Work out the finished part from the listing and answer in its coordinate system (mm). Round coordinates to 2 decimals unless told otherwise and drop trailing zeros. Order: outer loops, then holes, each group sorted by start corner. A loop starts at its lowest first (then second) coordinate and runs counter-clockwise, first axis right, second up. Notation, with made-up numbers: (60.25, -6.75) - (83.25, -6.75) arc R5 cw to (83.25, 1.25) - close; hole circle Ø11 at (11.5, 71.25). An arc over 180 degrees is marked (long way). Use CSV: the item, a comma, the result in double quotes.
from build123d import *

# Parameters (mm, degrees)
F0_W     = 78.734032
F0_H     = 94.131536
F1_DEPTH = 85.5


with BuildPart() as f1:
    # F0 (on Front) → F1 (new body)
    with BuildSketch(Plane.XZ):
        Rectangle(F0_W, F0_H)
    extrude(amount=F1_DEPTH)


with BuildPart() as f3:
    # F2 (on Front) → F3 (revolve)
    with BuildSketch(Plane.XZ):
        with BuildLine():
            Line((0, 0), (0, 49.300977))
            ThreePointArc((0, 49.300977), (-49.300977, 0), (0, -49.300977))
            Line((0, -49.300977), (0, 0))
        make_face()
    revolve(axis=Axis((0, 0, 0), (0, 0, -1)))


with BuildPart() as f1_1:
    add(f1.part)

    # F4: intersect F3
    add(f3.part, mode=Mode.INTERSECT)


solid = f1_1.part
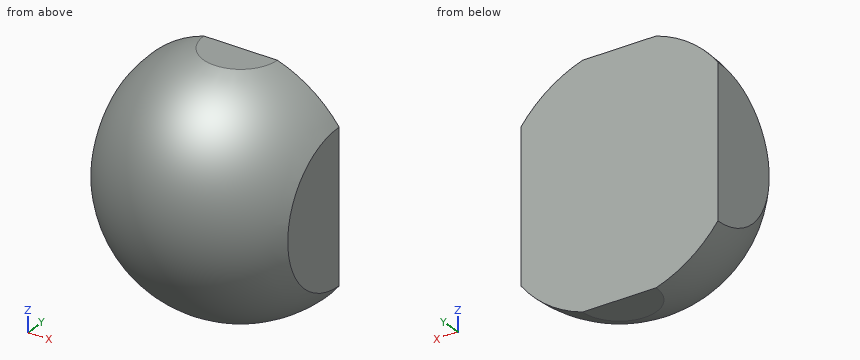
(1) Find section B-B (z = -15). Determine the outline of the cut face in (x, y), and give its area (3 significant figures).
Findings below:
outline,"(-39.37, -25.61) arc R46.96 ccw to (39.37, -25.61) - (39.37, 0) - (-39.37, 0) - close"
area,"3,200 mm²"
(2) Each of these flat-tipped pins is pushed along its axis until it touches: pin 1 (2 mm diameter, centred on y = -42, z = -0.5, fed in from +X); pin 2 (5 mm diameter, centred on x = 25.5, y = -29, fed in from -Z); pin 3 (2 mm diameter, centred on y = -35.5, z = 20.5, fed in from +X). Where does it stop, or does it pass through?
Findings below:
pin 1,"stops at x = 27.37"
pin 2,"stops at z = -33.56"
pin 3,"stops at x = 28.83"
(3) Find the intervals of material crossed by L1, parallel to Z at x = -20, y = -8; L2, parallel to Y at x = 35.5, z = -28; L3, parallel to Y at x = 22, z = -40, in increasing order. Write a range as from..to.
Findings below:
L1,"z = -44.35..44.35"
L2,"y = -19.66..0"
L3,"y = -18.62..0"
(4) Find section A-A (y = -6.5). Determine the outline of the cut face in (x, z).
Findings below:
outline,"(-39.37, -28.96) arc R48.87 ccw to (-13.16, -47.07) - (13.16, -47.07) arc R48.87 ccw to (39.37, -28.96) - (39.37, 28.96) arc R48.87 ccw to (13.16, 47.07) - (-13.16, 47.07) arc R48.87 ccw to (-39.37, 28.96) - close"
(5) Find section D-D (y = -45). Determine the outline of the cut face in (x, z), and give its area (3 significant figures).
Findings below:
outline,"circle Ø40.28 at (0, 0)"
area,"1,270 mm²"
(6) Find section C-C (x = 31). Determine the outline of the cut face in (y, z), and give its area (3 significant figures).
Findings below:
outline,"(0, -38.34) - (0, 38.34) arc R38.34 ccw to start"
area,"2,310 mm²"
